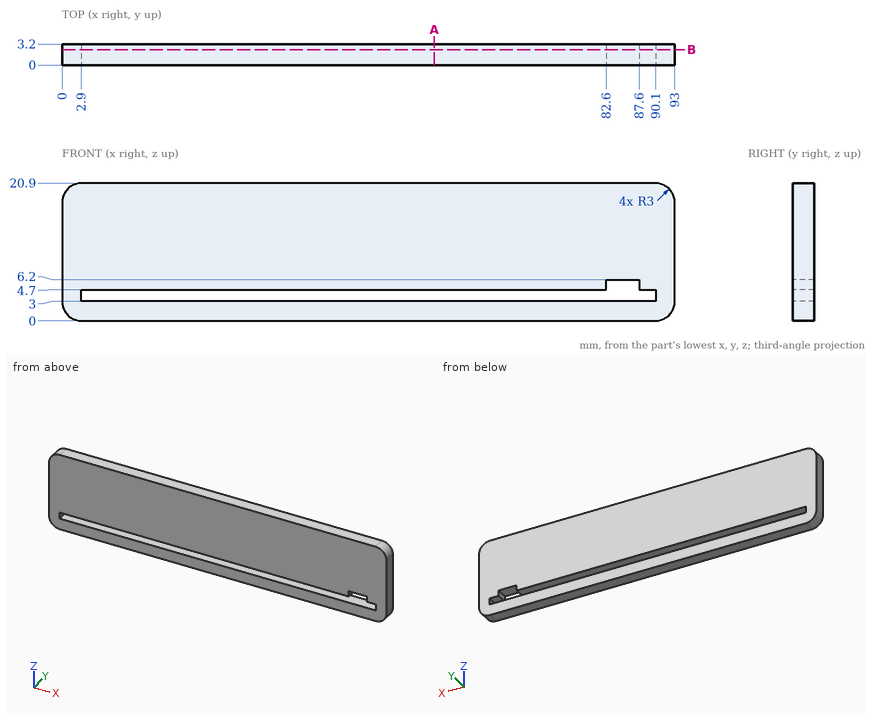
Input: dimensioned drawing with shaded views. Units: mm. Origin: part minimum x, y, z. Coordinates: 2 decimals unless noted, no trailing zeros. Loops run counter-clockwise (first coordinate to the right, second up) from the corner with the lowest first, then second, coordinate; pieces in that order, holes last. Notation, with made-up numbers: M 35.5,67 L 66.5,67 A27 cw 66.5,94 Z; hole C 42,7 d5. An arc over 180 degrees is marked long. Put each result on its own line as item: value.
(1) Cut plane B-B on y = 2.35. Return the cut outline in (x, z), then the cut area to 3 significant figures.
Answer sheet:
outline: M 0,3 A3 ccw 3,0 L 90,0 A3 ccw 93,3 L 93,17.9 A3 ccw 90,20.9 L 3,20.9 A3 ccw 0,17.9 Z; hole M 2.9,3 L 90.1,3 L 90.1,4.7 L 87.6,4.7 L 87.6,6.2 L 82.6,6.2 L 82.6,4.7 L 2.9,4.7 Z
area: 1,780 mm^2
(2) Material intervals for probe 1 along Z at (x, y) = (86, 1.6); probe 2 along Z at (x, y) = (69, 1.15); probe 3 along X at (y, z) = (0.55, 4.25), sorted ascending.
Answer sheet:
probe 1: z = 0 to 3, 6.2 to 20.9
probe 2: z = 0 to 3, 4.7 to 20.9
probe 3: x = 0 to 2.9, 90.1 to 93
(3) Cut plane A-A on x = 56.5. Return the cut outline in (y, z).
Answer sheet:
outline: M 0,0 L 3.2,0 L 3.2,3 L 0,3 Z; M 0,4.7 L 3.2,4.7 L 3.2,20.9 L 0,20.9 Z
